Here's how the part is built. I have some questions about the finished solid (model axes, mm). A direction names the side the tool comes from. Coordinates: 2 decimals unless noted, no trailing zeros. Write each loop counter-clockwise with the first axis right and the second up, starting at its lowest first coordinate (ties: lowest second). Pieces come first, ordered by that corner, then holes.
```python
from build123d import *

# Parameters (mm, degrees)
BOX006_W               = 6
BOX006_H               = 20
BOX006_DEPTH           = 2
CYLINDER022_R          = 8.85
CYLINDER022_DEPTH      = 15
CYLINDER019_R          = 1.35
CYLINDER019_DEPTH      = 5
CYLINDER002_R          = 3
CYLINDER002_DEPTH      = 3
CYLINDER018_R          = 8.85
CYLINDER018_DEPTH      = 13
CYLINDER017_R          = 9.75
CYLINDER017_DEPTH      = 13
BOX_W                  = 6
BOX_H                  = 5.5
BOX_DEPTH              = 3
BOX_PLACEMENT_ANGLE    = 135
BOX005_W               = 1
BOX005_H               = 1.5
BOX005_DEPTH           = 7.7
BOX004_W               = 1
BOX004_H               = 1.5
BOX004_DEPTH           = 7.7
FILLET003_R            = 1
BOX015_W               = 3
BOX015_H               = 3
BOX015_DEPTH           = 2.8
BOX016_W               = 3
BOX016_H               = 3.1
BOX016_DEPTH           = 2.8
BOX014_W               = 3
BOX014_H               = 3
BOX014_DEPTH           = 2.8
BOX013_W               = 3
BOX013_H               = 3
BOX013_DEPTH           = 2.8
BOX012_W               = 3
BOX012_H               = 3.1
BOX012_DEPTH           = 2.8
BOX011_W               = 3
BOX011_H               = 3
BOX011_DEPTH           = 2.8
BOX010_W               = 3
BOX010_H               = 3
BOX010_DEPTH           = 2.8
BOX009_W               = 3
BOX009_H               = 3
BOX009_DEPTH           = 2.8
BOX009_PLACEMENT_ANGLE = 45
BOX017_W               = 3
BOX017_H               = 3
BOX017_DEPTH           = 2.8
CYLINDER044_R          = 9
CYLINDER044_DEPTH      = 2.6
CYLINDER001_R          = 2
CYLINDER001_DEPTH      = 10.5
FILLET_R               = 1


with BuildPart() as cube006:
    # Box006 → Box006 (new body)
    with BuildSketch(Plane(origin=(-3, -10, -3), x_dir=(1, 0, 0), z_dir=(0, 0, 1))):
        with Locations((3, 10)):
            Rectangle(BOX006_W, BOX006_H)
    extrude(amount=BOX006_DEPTH)


with BuildPart() as cylinder022:
    # Cylinder022 → Cylinder022 (new body)
    with BuildSketch(Plane.XY.offset(-6)):
        Circle(CYLINDER022_R)
    extrude(amount=CYLINDER022_DEPTH)


with BuildPart() as cylinder019:
    # Cylinder019 → Cylinder019 (new body)
    with BuildSketch(Plane(origin=(-10.002388, 10.002388, 0), x_dir=(0, -1, 0), z_dir=(0, 0, 1))):
        Circle(CYLINDER019_R)
    extrude(amount=CYLINDER019_DEPTH)


with BuildPart() as obj1:
    # Cylinder002 → Cylinder002 (new body)
    with BuildSketch(Plane(origin=(-10.002388, 10.002388, 0), x_dir=(0, -1, 0), z_dir=(0, 0, 1))):
        Circle(CYLINDER002_R)
    extrude(amount=CYLINDER002_DEPTH)


with BuildPart() as negative:
    # Cylinder018 → Cylinder018 (new body)
    with BuildSketch(Plane.XY.offset(-5)):
        Circle(CYLINDER018_R)
    extrude(amount=CYLINDER018_DEPTH)


with BuildPart() as outer_wall:
    # Cylinder017 → Cylinder017 (new body)
    with BuildSketch(Plane.XY.offset(-5)):
        Circle(CYLINDER017_R)
    extrude(amount=CYLINDER017_DEPTH)

    # Cut008: cut Negative
    add(negative.part, mode=Mode.SUBTRACT)


with BuildPart() as connect:
    # Box → Box (new body)
    with BuildSketch(Plane.XY):
        with Locations((3, 2.75)):
            Rectangle(BOX_W, BOX_H)
    extrude(amount=BOX_DEPTH)


with BuildPart() as connect_1:
    # Box placement: moved
    add(connect.part.moved(Location((-3.005204, 6.894291, 0))).rotate(Axis((-3.005204, 6.894291, 0), (0, 0, 1)), BOX_PLACEMENT_ANGLE))

    # Fusion008: union obj1, Outer Wall
    add(obj1.part)
    add(outer_wall.part)

    # Cut: cut Cylinder019
    add(cylinder019.part, mode=Mode.SUBTRACT)

    # Cut009: cut Cylinder022
    add(cylinder022.part, mode=Mode.SUBTRACT)


with BuildPart() as cube005:
    # Box005 → Box005 (new body)
    with BuildSketch(Plane(origin=(-8, 0.75, -3.5), x_dir=(-1, 0, 0), z_dir=(0, 0, 1))):
        with Locations((0.5, 0.75)):
            Rectangle(BOX005_W, BOX005_H)
    extrude(amount=BOX005_DEPTH)


with BuildPart() as fillet003:
    # Box004 → Box004 (new body)
    with BuildSketch(Plane(origin=(8, -0.75, -3.5), x_dir=(1, 0, 0), z_dir=(0, 0, 1))):
        with Locations((0.5, 0.75)):
            Rectangle(BOX004_W, BOX004_H)
    extrude(amount=BOX004_DEPTH)

    # Fusion: union Cube005
    add(cube005.part)

    # Fusion024: union Connect
    add(connect_1.part)

    # Cut013012: cut Cube006
    add(cube006.part, mode=Mode.SUBTRACT)

    # Fillet003
    fillet003_edges = [fillet003.edges().sort_by_distance(p)[0] for p in [
        (-6.894291, 6.894291, 0),
        (-4.669835, 8.558922, 1.5),
        (-8.558922, 4.669835, 1.5),
    ]]
    fillet(fillet003_edges, radius=FILLET003_R)


with BuildPart() as cube015:
    # Box015 → Box015 (new body)
    with BuildSketch(Plane(origin=(3.7, 1.5, 2.6), x_dir=(1, 0, 0), z_dir=(0, 0, 1))):
        with Locations((1.5, 1.5)):
            Rectangle(BOX015_W, BOX015_H)
    extrude(amount=BOX015_DEPTH)


with BuildPart() as cube016:
    # Box016 → Box016 (new body)
    with BuildSketch(Plane(origin=(3, -1.55, 2.6), x_dir=(1, 0, 0), z_dir=(0, 0, 1))):
        with Locations((1.5, 1.55)):
            Rectangle(BOX016_W, BOX016_H)
    extrude(amount=BOX016_DEPTH)


with BuildPart() as fusion027:
    # Box014 → Box014 (new body)
    with BuildSketch(Plane(origin=(0.75, 2.4, 2.6), x_dir=(1, 0, 0), z_dir=(0, 0, 1))):
        with Locations((1.5, 1.5)):
            Rectangle(BOX014_W, BOX014_H)
    extrude(amount=BOX014_DEPTH)

    # Fusion027: union Cube015, Cube016
    add(cube015.part)
    add(cube016.part)


with BuildPart() as cube013:
    # Box013 → Box013 (new body)
    with BuildSketch(Plane(origin=(-6.7, 1.5, 2.6), x_dir=(1, 0, 0), z_dir=(0, 0, 1))):
        with Locations((1.5, 1.5)):
            Rectangle(BOX013_W, BOX013_H)
    extrude(amount=BOX013_DEPTH)


with BuildPart() as cube012:
    # Box012 → Box012 (new body)
    with BuildSketch(Plane(origin=(-6, -1.55, 2.6), x_dir=(1, 0, 0), z_dir=(0, 0, 1))):
        with Locations((1.5, 1.55)):
            Rectangle(BOX012_W, BOX012_H)
    extrude(amount=BOX012_DEPTH)


with BuildPart() as cube011:
    # Box011 → Box011 (new body)
    with BuildSketch(Plane(origin=(-6.7, -4.5, 2.6), x_dir=(1, 0, 0), z_dir=(0, 0, 1))):
        with Locations((1.5, 1.5)):
            Rectangle(BOX011_W, BOX011_H)
    extrude(amount=BOX011_DEPTH)


with BuildPart() as cube010:
    # Box010 → Box010 (new body)
    with BuildSketch(Plane(origin=(-3.75, -5.4, 2.6), x_dir=(1, 0, 0), z_dir=(0, 0, 1))):
        with Locations((1.5, 1.5)):
            Rectangle(BOX010_W, BOX010_H)
    extrude(amount=BOX010_DEPTH)


with BuildPart() as cube009:
    # Box009 → Box009 (new body)
    with BuildSketch(Plane.XY):
        with Locations((1.5, 1.5)):
            Rectangle(BOX009_W, BOX009_H)
    extrude(amount=BOX009_DEPTH)


with BuildPart() as cube009_1:
    # Box009 placement: moved
    add(cube009.part.moved(Location((-0.15, -8.06, 2.6))).rotate(Axis((-0.15, -8.06, 2.6), (0, 0, 1)), BOX009_PLACEMENT_ANGLE))


with BuildPart() as compound:
    # Box017 → Box017 (new body)
    with BuildSketch(Plane(origin=(-3.75, 2.4, 2.6), x_dir=(1, 0, 0), z_dir=(0, 0, 1))):
        with Locations((1.5, 1.5)):
            Rectangle(BOX017_W, BOX017_H)
    extrude(amount=BOX017_DEPTH)

    # Fusion026: union Cube013, Cube012, Cube011, Cube010, Cube009
    add(cube013.part)
    add(cube012.part)
    add(cube011.part)
    add(cube010.part)
    add(cube009_1.part)

    # Compound: union Fusion027
    add(fusion027.part)


with BuildPart() as cut013013:
    # Cylinder044 → Cylinder044 (new body)
    with BuildSketch(Plane.XY.offset(2.7)):
        Circle(CYLINDER044_R)
    extrude(amount=CYLINDER044_DEPTH)

    # Cut013013: cut Compound
    add(compound.part, mode=Mode.SUBTRACT)


with BuildPart() as connector_base:
    # Cylinder001 → Cylinder001 (new body)
    with BuildSketch(Plane.XY.offset(4)):
        Circle(CYLINDER001_R)
    extrude(amount=CYLINDER001_DEPTH)

    # Fillet
    fillet_edges = [connector_base.edges().sort_by_distance(p)[0] for p in [
        (-2, 0, 14.5),
    ]]
    fillet(fillet_edges, radius=FILLET_R)

    # Fusion023: union Cut013013
    add(cut013013.part)

    # Fusion025: union Fillet003
    add(fillet003.part)


with BuildPart() as connector_base_1:
    # Fusion025 placement: moved
    add(connector_base.part.moved(Location((0, 0, 10))))


solid = connector_base_1.part
```
1) Imagine slicing it at B-B on y = -7.25. Please give me the cut outline in (x, z).
Values follow:
outline: (-6.52, 5) - (-5.08, 5) - (-5.08, 12.7) - (-0.96, 12.7) - (-0.96, 15.3) - (-5.08, 15.3) - (-5.08, 18) - (-6.52, 18) - close; (0.66, 12.7) - (5.08, 12.7) - (5.08, 5) - (6.52, 5) - (6.52, 18) - (5.08, 18) - (5.08, 15.3) - (0.66, 15.3) - close
2) Imagine slicing it at A-A on z = 8.5. Please give me the cut outline in (x, y).
Values follow:
outline: (-8.82, -0.75) - (-8, -0.75) - (-8, 0.75) - (-8.82, 0.75) arc R8.85 cw to (-3, 8.33) - (-3, 9.28) arc R9.75 ccw to (-3, -9.28) - (-3, -8.33) arc R8.85 cw to start; (3, -9.28) arc R9.75 ccw to (3, 9.28) - (3, 8.33) arc R8.85 cw to (8.82, 0.75) - (8, 0.75) - (8, -0.75) - (8.82, -0.75) arc R8.85 cw to (3, -8.33) - close
3) We'd pull the mould along Y, two halves only. Please class faces 5 (the face through (8.4, 0, 6.5)), 6 (the face through (3, -9, 8)), 7 (the face through (-1.2, -7.01, 13.98)): pulls with the +Y half, pulls with the -Y half, needs draft (parallel to the pull), parting line crosses it, or undercut.
Values follow:
face 5: undercut
face 6: needs draft
face 7: undercut
4) On a 3-axis mill with a long thin cutter (end or side, diameter ignored), from which of +Z, -Z, +X, -X, +Y, -Y can I reach the whole of each face in a straight line? I mean faces 1 (the face through (-3.75, -5, 14)), 2 (the face through (-10.07, 6.18, 11.45)), 3 (the face through (-8.4, 0.75, 9.6)), 4 (the face through (0, -2, 19)). Say none if no direction works.
Values follow:
face 1: +Z, -Z
face 2: +Z, -Z, -X
face 3: -Z
face 4: +Z
5) I need wall thicknesses on probe 1 along Y at (x, z) = (0, 17.1); probe 2 along X at (y, z) = (-3, 12); probe 3 along Z at (x, y) = (2.25, -1). Which ranges of each line are inside material? Lowest first, please.
Values follow:
probe 1: y = -9.75 to -8.85, -2 to 2, 8.85 to 9.75
probe 2: x = -9.28 to -8.33, 8.33 to 9.28
probe 3: z = 12.7 to 15.3
6) Imagine slicing it at C-C on z = 14. Count the separate pieces of the cut face and the enclosed holes in it, then the cut area to 3 significant figures.
Values follow:
separate pieces: 1
enclosed holes: 2
area: 218 mm2
7) Will these pins go through, and if not, where does the flat tip stop? pin 1 (1 mm diameter, centred on x = -2, z = 7, fed in from +Y); pin 2 (5 mm diameter, centred on y = 10, z = 8, fed in from +X); pin 3 (6 mm diameter, centred on x = -5, z = 15, fed in from -Y).
Values follow:
pin 1: stops at y = 9.63
pin 2: stops at x = 6.23
pin 3: stops at y = -9.54
